Input: part model. Units: mm. Frame: model coordinates. Face numbers are marked on the shaded views. A direction names the side the tool comes from. Coordinates: 2 decimals unless noted, no trailing zeros. Write each loop counter-clockwise with the first axis right and the second up, starting at its lowest first coordinate (ties: lowest second). Pieces come first, ordered by that corner, then holes.
1) Section query B-B (z = 0). State how many separate pieces and enclosed holes the cut face has, then the cut area to 3 significant figures.
2) Set-up query: the marked faces 1 and 2. Return all of +Z, -Z, +X, -X, +Y, -Y with unobstructed straight access to the full face (end or side cutting, diameter ignored); none if empty.
3) Line query: L1, parallel to Z at x = 1, y = 17; L2, parallel to Z at x = 1.3, y = 17.5; L3, parallel to X at y = 30.5, z = -4.5. Output: solid intervals per line, ascending.
4) Section query A-A (x = 27.5). Output: boundary loops of the cut face in (y, z), then the cut area to 3 significant figures.
5) Section query D-D (x = 8). Output: boundary loops of the cut face in (y, z).
6) Pin query (flat end, axial travel): pin 1 Ø5.5 at (y, z) = (35, 0) entering from -X; pin 2 Ø8 at (x, y) = (4.5, -28) entering from -Z; pin 3 Ø3 at (x, y) = (20.5, -22.5) entering from +Z; pin 4 Ø5 at (x, z) = (6, -11.5) entering from +Y. Return the tip coordinate at first contact, or that it passes through.
from build123d import *

# Parameters (mm, degrees)
SKETCH2_R                         = 25
BOSS_EXTRUDE1_DEPTH               = 7.7
SKETCH3_R                         = 25
BOSS_EXTRUDE2_DEPTH               = 0.3
BOSS_EXTRUDE2_TAPER               = 44.999999949
SKETCH4_R                         = 24
BOSS_EXTRUDE3_DEPTH               = 19.5
SKETCH5_R                         = 22.741139955
BOSS_EXTRUDE4_DEPTH               = 2.5
BOSS_EXTRUDE4_TAPER               = 15.02708836
F_6_0_6_DIAMETER_HOLE1_AT_2_COUNT = 2
F_6_0_6_DIAMETER_HOLE1_AT_2_PITCH = 35
F_6_0_6_DIAMETER_HOLE1_AT_3_COUNT = 2
F_6_0_6_DIAMETER_HOLE1_AT_3_PITCH = 60.621778265
F_6_0_6_DIAMETER_HOLE1_AT_4_COUNT = 2
F_6_0_6_DIAMETER_HOLE1_AT_4_PITCH = 70
F_6_0_6_DIAMETER_HOLE1_AT_5_COUNT = 2
F_6_0_6_DIAMETER_HOLE1_AT_5_PITCH = 60.621778265
F_6_0_6_DIAMETER_HOLE1_AT_6_COUNT = 2
F_6_0_6_DIAMETER_HOLE1_AT_6_PITCH = 35
CHAMFER1_SIZE                     = 0.3
FILLET1_R                         = 0.5
FILLET2_R                         = 1


with BuildPart() as part:
    # Sketch1 → Revolve1 (revolve)
    with BuildSketch(Plane.XY):
        with BuildLine():
            Line((0, 41), (0, 0))
            Line((0, 0), (5, 0))
            Line((5, 0), (5, 25))
            ThreePointArc((5, 25), (3.585786438, 25.585786438), (3, 27))
            Line((3, 27), (3, 41))
            Line((3, 41), (0, 41))
        make_face()
    revolve(axis=Axis((0, 0, 0), (1, 0, 0)))

    # Sketch2 → Boss-Extrude1 (add)
    with BuildSketch(Plane(origin=(5, 0, 0), x_dir=(0, 0, -1), z_dir=(1, 0, 0))):
        Circle(SKETCH2_R)
    extrude(amount=BOSS_EXTRUDE1_DEPTH)

    # Sketch3 → Boss-Extrude2 (add)
    with BuildSketch(Plane(origin=(12.7, 0, 0), x_dir=(0, 0, -1), z_dir=(1, 0, 0))):
        Circle(SKETCH3_R)
    extrude(amount=BOSS_EXTRUDE2_DEPTH, taper=BOSS_EXTRUDE2_TAPER)

    # Sketch4 → Boss-Extrude3 (add)
    with BuildSketch(Plane(origin=(13, 0, 0), x_dir=(0, 0, -1), z_dir=(1, 0, 0))):
        Circle(SKETCH4_R)
    extrude(amount=BOSS_EXTRUDE3_DEPTH)

    # Sketch5 → Boss-Extrude4 (add)
    with BuildSketch(Plane(origin=(32.5, 0, 0), x_dir=(0, 0, -1), z_dir=(1, 0, 0))):
        Circle(SKETCH5_R)
    extrude(amount=BOSS_EXTRUDE4_DEPTH, taper=BOSS_EXTRUDE4_TAPER)

    # Sketch6 → Ø6.0 (6) Diameter Hole1 (revolve, cut)
    with BuildSketch(Plane(origin=(3, -17.5, 30.310889132), x_dir=(0, 0, -1), z_dir=(0, 1, 0))):
        Polygon((0, 0), (0, 3), (3, 3), (3, 0.326896118), (3.326896118, 0), align=None)
    f_6_0_6_diameter_hole1 = revolve(axis=Axis((9.35, -17.5, 30.310889132), (-1, 0, 0)), mode=Mode.SUBTRACT)

    # Ø6.0 (6) Diameter Hole1 at 2: Ø6.0 (6) Diameter Hole1 ×2
    with Locations(*[(0, i * F_6_0_6_DIAMETER_HOLE1_AT_2_PITCH, 0) for i in range(1, F_6_0_6_DIAMETER_HOLE1_AT_2_COUNT)]):
        add(f_6_0_6_diameter_hole1, mode=Mode.SUBTRACT)

    # Ø6.0 (6) Diameter Hole1 at 3: Ø6.0 (6) Diameter Hole1 ×2
    with Locations(*[Vector(0, 0.866025404, -0.5) * (i * F_6_0_6_DIAMETER_HOLE1_AT_3_PITCH) for i in range(1, F_6_0_6_DIAMETER_HOLE1_AT_3_COUNT)]):
        add(f_6_0_6_diameter_hole1, mode=Mode.SUBTRACT)

    # Ø6.0 (6) Diameter Hole1 at 4: Ø6.0 (6) Diameter Hole1 ×2
    with Locations(*[Vector(0, 0.5, -0.866025404) * (i * F_6_0_6_DIAMETER_HOLE1_AT_4_PITCH) for i in range(1, F_6_0_6_DIAMETER_HOLE1_AT_4_COUNT)]):
        add(f_6_0_6_diameter_hole1, mode=Mode.SUBTRACT)

    # Ø6.0 (6) Diameter Hole1 at 5: Ø6.0 (6) Diameter Hole1 ×2
    with Locations(*[(0, 0, -i * F_6_0_6_DIAMETER_HOLE1_AT_5_PITCH) for i in range(1, F_6_0_6_DIAMETER_HOLE1_AT_5_COUNT)]):
        add(f_6_0_6_diameter_hole1, mode=Mode.SUBTRACT)

    # Ø6.0 (6) Diameter Hole1 at 6: Ø6.0 (6) Diameter Hole1 ×2
    with Locations(*[Vector(0, -0.5, -0.866025404) * (i * F_6_0_6_DIAMETER_HOLE1_AT_6_PITCH) for i in range(1, F_6_0_6_DIAMETER_HOLE1_AT_6_COUNT)]):
        add(f_6_0_6_diameter_hole1, mode=Mode.SUBTRACT)

    # Chamfer1
    chamfer1_edges = [part.edges().sort_by_distance(p)[0] for p in [
        (0, -35, 3),
        (0, -17.5, -27.310889132),
        (0, 17.5, -27.310889132),
        (0, -41, 0),
        (0, 35, 3),
        (0, 17.5, 33.310889132),
        (0, -17.5, 33.310889132),
        (3, -41, 0),
    ]]
    chamfer(chamfer1_edges, length=CHAMFER1_SIZE)

    # Fillet1
    fillet1_edges = [part.edges().sort_by_distance(p)[0] for p in [
        (32.5, 0, 22.741139955),
    ]]
    fillet(fillet1_edges, radius=FILLET1_R)

    # Fillet2
    fillet2_edges = [part.edges().sort_by_distance(p)[0] for p in [
        (35, 0, 22.07),
    ]]
    fillet(fillet2_edges, radius=FILLET2_R)


solid = part.part
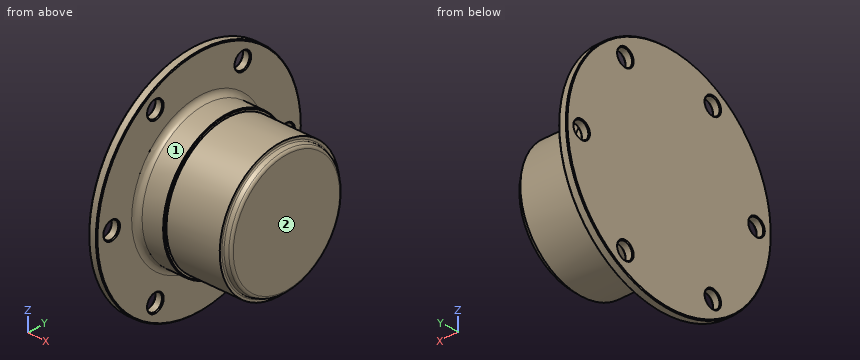
Answer:
1. separate pieces: 3
1. enclosed holes: 0
1. area: 1,760 mm2
2. face 1: +X
2. face 2: +Z, -Z, +X, +Y, -Y
3. L1: z = -37.31 to -33.27, -27.35 to 27.35, 33.27 to 37.31
3. L2: z = -37.08 to -33.31, -27.31 to 27.31, 33.31 to 37.08
3. L3: x = 0 to 3
4. outline: circle Ø48 at (0, 0)
4. area: 1,810 mm2
5. outline: circle Ø50 at (0, 0)
6. pin 1: passes through
6. pin 2: stops at z = -32.93
6. pin 3: stops at z = 11.62
6. pin 4: stops at y = 23.32
